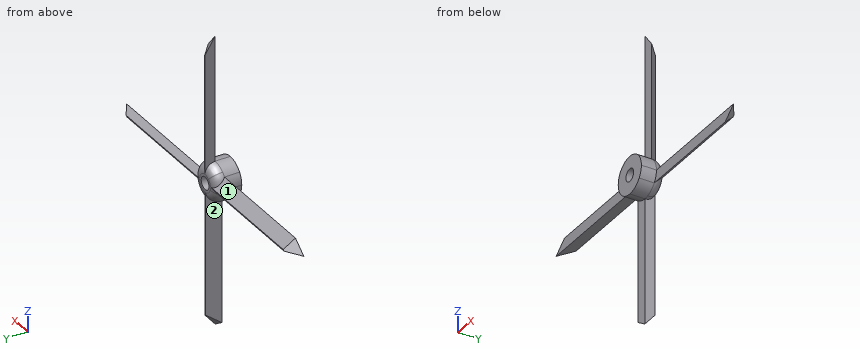
from build123d import *

# Parameters (mm, degrees)
F0_R         = 3.175
F1_DEPTH     = 12.7
F2_DEPTH     = 5.08
F3_SIZE      = 5.07999
F4_T3_ANGLE  = 206.8900819295
F4_T7_ANGLE  = 130.484631046
F4_T11_ANGLE = 206.8900819295
F4_T15_ANGLE = 206.8900819295
F4_T19_ANGLE = 130.484631046
F4_T23_ANGLE = 206.8900819295
F4_T27_ANGLE = 206.8900819295
F4_T31_ANGLE = 130.484631046
F4_T35_ANGLE = 206.8900819295
F4_T39_ANGLE = 206.8900819295
F4_T43_ANGLE = 130.484631046
F4_T47_ANGLE = 206.8900819295


# Not quite as in the source:
# - a fillet or chamfer that OpenCascade refuses, or shapes differently, is made with other operations: its cross-section is extruded or revolved along the edge and cut away or added
# - a fillet or chamfer is up to 0.001 mm smaller than in the source, because OpenCascade refuses the exact size


with BuildPart() as f1:
    # F0 (on Front) → F1 (new body)
    with BuildSketch(Plane.XZ):
        with BuildLine():
            ThreePointArc((15.8353851332, 8.5368495443), (17.1826135049, 11.1877228091), (17.6467685365, 14.1248495443))
            ThreePointArc((17.6467685365, 14.1248495443), (16.6056156886, 18.4549722331), (13.7097685365, 21.838466141))
            ThreePointArc((13.7097685365, 21.838466141), (11.0588952717, 23.1856945127), (8.1217685365, 23.6498495443))
            ThreePointArc((8.1217685365, 23.6498495443), (3.7916458477, 22.6086966964), (0.4081519399, 19.7128495443))
            ThreePointArc((0.4081519399, 19.7128495443), (-0.9390764319, 17.0619762795), (-1.4032314635, 14.1248495443))
            ThreePointArc((-1.4032314635, 14.1248495443), (-0.3620786156, 9.7947268555), (2.5337685365, 6.4112329477))
            ThreePointArc((2.5337685365, 6.4112329477), (5.1846418013, 5.0640045759), (8.1217685365, 4.5998495443))
            ThreePointArc((8.1217685365, 4.5998495443), (12.4518912253, 5.6410023922), (15.8353851332, 8.5368495443))
        make_face()
        with Locations((8.1217685365, 14.1248495443)):
            Circle(F0_R, mode=Mode.SUBTRACT)
    extrude(amount=F1_DEPTH)

    # F0 (on Front) → F2 (join)
    with BuildSketch(Plane.XZ):
        with BuildLine():
            ThreePointArc((8.1217685365, 23.6498495443), (11.0588952717, 23.1856945127), (13.7097685365, 21.838466141))
            Line((13.7097685365, 21.838466141), (13.7097685365, 80.258466141))
            Line((13.7097685365, 80.258466141), (8.1217685365, 87.1498495443))
            Line((8.1217685365, 87.1498495443), (8.1217685365, 23.6498495443))
        make_face()
        with BuildLine():
            Line((81.1467685365, 14.1248495443), (17.6467685365, 14.1248495443))
            ThreePointArc((17.6467685365, 14.1248495443), (17.1826135049, 11.1877228091), (15.8353851332, 8.5368495443))
            Line((15.8353851332, 8.5368495443), (74.2553851332, 8.5368495443))
            Line((74.2553851332, 8.5368495443), (81.1467685365, 14.1248495443))
        make_face()
        with BuildLine():
            ThreePointArc((-1.4032314635, 14.1248495443), (-0.9390764319, 17.0619762795), (0.4081519399, 19.7128495443))
            Line((0.4081519399, 19.7128495443), (-58.0118480601, 19.7128495443))
            Line((-58.0118480601, 19.7128495443), (-64.9032314635, 14.1248495443))
            Line((-64.9032314635, 14.1248495443), (-1.4032314635, 14.1248495443))
        make_face()
        with BuildLine():
            Line((8.1217685365, -58.9001504557), (8.1217685365, 4.5998495443))
            ThreePointArc((8.1217685365, 4.5998495443), (5.1846418013, 5.0640045759), (2.5337685365, 6.4112329477))
            Line((2.5337685365, 6.4112329477), (2.5337685365, -55.2206523716))
            Line((2.5337685365, -55.2206523716), (8.1217685365, -58.9001504557))
        make_face()
    extrude(amount=F2_DEPTH)

    # F3 (size 5.08 in the source; OpenCascade refuses exactly that, so slightly less here)
    f3_edges = [f1.edges().sort_by_distance(p)[0] for p in [
        (77.701077, 0, 11.33085),
        (45.045385, 0, 8.53685),
        (13.709769, 0, 51.048466),
        (10.915769, 0, 83.704158),
        (2.533769, 0, -24.40471),
        (5.327769, 0, -57.060401),
        (-28.801848, 0, 19.71285),
        (-61.45754, 0, 16.91885),
    ]]
    chamfer(f3_edges, length=F3_SIZE)

    # F4: fillet of radius 5.08 on 4 edges, made by hand


with BuildPart() as f4_tool1:
    # F4_s2 → F4_t3 (revolve)
    with BuildSketch(Plane(origin=(10.9000788328, 0, 2.6359089402), x_dir=(0, 1, 0), z_dir=(-0.9719833666, 0, -0.2350496437))):
        with BuildLine():
            ThreePointArc((-5.08, -2.2951000126), (-1.4878975516, -3.7829975641), (0, -7.3751000126))
            Line((0, -7.3751000126), (0, -2.2951000126))
            Line((0, -2.2951000126), (-5.08, -2.2951000126))
        make_face()
    revolve(axis=Axis((8.1217685365, 0, 14.1248495443), (0, -1, 0)), revolution_arc=F4_T3_ANGLE)

    split(bisect_by=Plane(origin=(0, -6.8084197722, 6.8084197722), x_dir=(1, 0, 0), z_dir=(0, 0.7071067812, -0.7071067812)), keep=Keep.TOP)


with BuildPart() as f4_tool5:
    # F4_s6 → F4_t7 (revolve)
    with BuildSketch(Plane.XY.offset(14.1248495443)):
        with BuildLine():
            ThreePointArc((17.6467685365, -5.08), (16.158870985, -1.4878975516), (12.5667685365, 0))
            Line((12.5667685365, 0), (17.6467685365, 0))
            Line((17.6467685365, 0), (17.6467685365, -5.08))
        make_face()
    revolve(axis=Axis((8.1217685365, 0, 14.1248495443), (0, -1, 0)), revolution_arc=F4_T7_ANGLE)

    split(bisect_by=Plane(origin=(4.3148892683, 4.3148892683, 0), x_dir=(0, 0, 1), z_dir=(0.7071067812, 0.7071067812, 0)), keep=Keep.TOP)


with BuildPart() as f4_tool9:
    # F4_s10 → F4_t11 (revolve)
    with BuildSketch(Plane(origin=(10.9000788328, 0, 2.6359089402), x_dir=(0, 1, 0), z_dir=(-0.9719833666, 0, -0.2350496437))):
        with BuildLine():
            ThreePointArc((-5.08, -2.2951000126), (-1.4878975516, -3.7829975641), (0, -7.3751000126))
            Line((0, -7.3751000126), (0, -2.2951000126))
            Line((0, -2.2951000126), (-5.08, -2.2951000126))
        make_face()
    revolve(axis=Axis((8.1217685365, 0, 14.1248495443), (0, -1, 0)), revolution_arc=F4_T11_ANGLE)

    split(bisect_by=Plane.YZ.offset(8.1217685365), keep=Keep.BOTTOM)


with BuildPart() as f4_tool13:
    # F4_s14 → F4_t15 (revolve)
    with BuildSketch(Plane(origin=(-2.7783102963, 0, 11.4889406041), x_dir=(0, 1, 0), z_dir=(-0.2350496437, 0, 0.9719833666))):
        with BuildLine():
            ThreePointArc((-5.08, -1.6892647777), (-1.4878975516, -3.1771623292), (0, -6.7692647777))
            Line((0, -6.7692647777), (0, -1.6892647777))
            Line((0, -1.6892647777), (-5.08, -1.6892647777))
        make_face()
    revolve(axis=Axis((8.1217685365, 0, 14.1248495443), (0, -1, 0)), revolution_arc=F4_T15_ANGLE)

    split(bisect_by=Plane(origin=(3.8068792683, -3.8068792683, 0), x_dir=(0, 0, 1), z_dir=(-0.7071067812, 0.7071067812, 0)), keep=Keep.TOP)


with BuildPart() as f4_tool17:
    # F4_s18 → F4_t19 (revolve)
    with BuildSketch(Plane.YZ.offset(8.1217685365)):
        with BuildLine():
            ThreePointArc((-5.08, 4.5998495443), (-1.4878975516, 6.0877470959), (0, 9.6798495443))
            Line((0, 9.6798495443), (0, 4.5998495443))
            Line((0, 4.5998495443), (-5.08, 4.5998495443))
        make_face()
    revolve(axis=Axis((8.1217685365, 0, 14.1248495443), (0, -1, 0)), revolution_arc=F4_T19_ANGLE)

    split(bisect_by=Plane(origin=(0, -6.8084197722, 6.8084197722), x_dir=(1, 0, 0), z_dir=(0, 0.7071067812, -0.7071067812)), keep=Keep.TOP)


with BuildPart() as f4_tool21:
    # F4_s22 → F4_t23 (revolve)
    with BuildSketch(Plane(origin=(-2.7783102963, 0, 11.4889406041), x_dir=(0, 1, 0), z_dir=(-0.2350496437, 0, 0.9719833666))):
        with BuildLine():
            ThreePointArc((-5.08, -1.6892647777), (-1.4878975516, -3.1771623292), (0, -6.7692647777))
            Line((0, -6.7692647777), (0, -1.6892647777))
            Line((0, -1.6892647777), (-5.08, -1.6892647777))
        make_face()
    revolve(axis=Axis((8.1217685365, 0, 14.1248495443), (0, -1, 0)), revolution_arc=F4_T23_ANGLE)

    split(bisect_by=Plane.XY.offset(14.1248495443), keep=Keep.TOP)


with BuildPart() as f4_tool25:
    # F4_s26 → F4_t27 (revolve)
    with BuildSketch(Plane(origin=(-2.7783102963, 0, 11.4889406041), x_dir=(0, 1, 0), z_dir=(0.2350496437, 0, -0.9719833666))):
        with BuildLine():
            ThreePointArc((-5.08, 20.7392647777), (-1.4878975516, 19.2513672261), (0, 15.6592647777))
            Line((0, 15.6592647777), (0, 20.7392647777))
            Line((0, 20.7392647777), (-5.08, 20.7392647777))
        make_face()
    revolve(axis=Axis((8.1217685365, 0, 14.1248495443), (0, -1, 0)), revolution_arc=F4_T27_ANGLE)

    split(bisect_by=Plane(origin=(4.3148892683, 4.3148892683, 0), x_dir=(0, 0, 1), z_dir=(0.7071067812, 0.7071067812, 0)), keep=Keep.TOP)


with BuildPart() as f4_tool29:
    # F4_s30 → F4_t31 (revolve)
    with BuildSketch(Plane.YZ.offset(8.1217685365)):
        with BuildLine():
            ThreePointArc((-5.08, 23.6498495443), (-1.4878975516, 22.1619519927), (0, 18.5698495443))
            Line((0, 18.5698495443), (0, 23.6498495443))
            Line((0, 23.6498495443), (-5.08, 23.6498495443))
        make_face()
    revolve(axis=Axis((8.1217685365, 0, 14.1248495443), (0, -1, 0)), revolution_arc=F4_T31_ANGLE)

    split(bisect_by=Plane(origin=(0, 7.3164297722, 7.3164297722), x_dir=(1, 0, 0), z_dir=(0, 0.7071067812, 0.7071067812)), keep=Keep.TOP)


with BuildPart() as f4_tool33:
    # F4_s34 → F4_t35 (revolve)
    with BuildSketch(Plane(origin=(-2.7783102963, 0, 11.4889406041), x_dir=(0, 1, 0), z_dir=(0.2350496437, 0, -0.9719833666))):
        with BuildLine():
            ThreePointArc((-5.08, 20.7392647777), (-1.4878975516, 19.2513672261), (0, 15.6592647777))
            Line((0, 15.6592647777), (0, 20.7392647777))
            Line((0, 20.7392647777), (-5.08, 20.7392647777))
        make_face()
    revolve(axis=Axis((8.1217685365, 0, 14.1248495443), (0, -1, 0)), revolution_arc=F4_T35_ANGLE)

    split(bisect_by=Plane.XY.offset(14.1248495443), keep=Keep.BOTTOM)


with BuildPart() as f4_tool37:
    # F4_s38 → F4_t39 (revolve)
    with BuildSketch(Plane(origin=(10.9000788328, 0, 2.6359089402), x_dir=(0, 1, 0), z_dir=(0.9719833666, 0, 0.2350496437))):
        with BuildLine():
            ThreePointArc((-5.08, 21.3451000126), (-1.4878975516, 19.857202461), (0, 16.2651000126))
            Line((0, 16.2651000126), (0, 21.3451000126))
            Line((0, 21.3451000126), (-5.08, 21.3451000126))
        make_face()
    revolve(axis=Axis((8.1217685365, 0, 14.1248495443), (0, -1, 0)), revolution_arc=F4_T39_ANGLE)

    split(bisect_by=Plane(origin=(0, 7.3164297722, 7.3164297722), x_dir=(1, 0, 0), z_dir=(0, 0.7071067812, 0.7071067812)), keep=Keep.TOP)


with BuildPart() as f4_tool41:
    # F4_s42 → F4_t43 (revolve)
    with BuildSketch(Plane.XY.offset(14.1248495443)):
        with BuildLine():
            ThreePointArc((-1.4032314635, -5.08), (0.0846660881, -1.4878975516), (3.6767685365, 0))
            Line((3.6767685365, 0), (-1.4032314635, 0))
            Line((-1.4032314635, 0), (-1.4032314635, -5.08))
        make_face()
    revolve(axis=Axis((8.1217685365, 0, 14.1248495443), (0, -1, 0)), revolution_arc=F4_T43_ANGLE)

    split(bisect_by=Plane(origin=(3.8068792683, -3.8068792683, 0), x_dir=(0, 0, 1), z_dir=(-0.7071067812, 0.7071067812, 0)), keep=Keep.TOP)


with BuildPart() as f4_tool45:
    # F4_s46 → F4_t47 (revolve)
    with BuildSketch(Plane(origin=(10.9000788328, 0, 2.6359089402), x_dir=(0, 1, 0), z_dir=(0.9719833666, 0, 0.2350496437))):
        with BuildLine():
            ThreePointArc((-5.08, 21.3451000126), (-1.4878975516, 19.857202461), (0, 16.2651000126))
            Line((0, 16.2651000126), (0, 21.3451000126))
            Line((0, 21.3451000126), (-5.08, 21.3451000126))
        make_face()
    revolve(axis=Axis((8.1217685365, 0, 14.1248495443), (0, -1, 0)), revolution_arc=F4_T47_ANGLE)

    split(bisect_by=Plane.YZ.offset(8.1217685365), keep=Keep.TOP)


with BuildPart() as f1_1:
    add(f1.part)

    # F4_t49: cut F4_tool1, F4_tool5, F4_tool9, F4_tool13, F4_tool17, F4_tool21, F4_tool25, F4_tool29, F4_tool33, F4_tool37, F4_tool41, F4_tool45
    add([f4_tool1.part, f4_tool5.part, f4_tool9.part, f4_tool13.part, f4_tool17.part, f4_tool21.part, f4_tool25.part, f4_tool29.part, f4_tool33.part, f4_tool37.part, f4_tool41.part, f4_tool45.part], mode=Mode.SUBTRACT)


solid = f1_1.part
Verification items for the finished model (mm, model axes). Face numbers are marked on the shaded views. Give positions to 0.01 mm unless a question says otherwise; leave off trailing zeros. Loops run counter-clockwise (first coordinate to the right, second up) from the corner with the lowest first, then second, coordinate; pieces in that order, holes last.
1. Material ranges on probe 1 along Z at (x, y) = (-46.5, -3); probe 2 along Z at (x, y) = (51.5, -5); probe 3 along Z at (x, y) = (7.5, -7.75), recorded low to high.
Derived:
probe 1: z = 14.12 to 17.63
probe 2: z = 8.62 to 14.12
probe 3: z = 4.62 to 11.01, 17.24 to 23.63
2. Go/stop test with flat-tipped pins: P1, Ø6, axis at x = 4.5, z = -41, coming from the -Y side; P2, Ø5, axis at x = -15.5, y = -5.5, coming from the -Z side; P3, Ø2, axis at x = 57.5, y = -5, coming from the +Z side. Record where each tip stops, or that it passes through.
Derived:
P1: stops at y = -5.08
P2: stops at z = 14.12
P3: stops at z = 14.12
3. Release check for a two-part mould opening along X. For the marked faces 1 and 2 record: +X half, -X half, draft (parallel to the pull), parting line (faces both ways), or undercut.
Derived:
face 1: draft
face 2: -X half
4. Cross-section at A-A on y = -9. Record the cut outline in (x, z) (3 decimals).
Derived:
outline: circle Ø19.05 at (8.122, 14.125); hole circle Ø6.35 at (8.122, 14.125)
